Build history of the part. All positions in model axes, mm. A direction names the side the tool comes from. Coordinates: 2 decimals unless noted, no trailing zeros. Write each loop counter-clockwise with the first axis right and the second up, starting at its lowest first coordinate (ties: lowest second). Pieces come first, ordered by that corner, then holes.
```python
from build123d import *

# Parameters (mm, degrees)
F0_R     = 35.394351
F1_DEPTH = 116.078
F2_R     = 31.583321
F3_DEPTH = 108.204
F4_DEPTH = 1.016
F5_W     = 28.326623
F5_H     = 68.561267
F6_DEPTH = 66.7


with BuildPart() as f1:
    # F0 (on Front) → F1 (new body)
    with BuildSketch(Plane.XZ):
        Circle(F0_R)
    extrude(amount=F1_DEPTH)

    # F2 (on Front) → F3 (cut)
    with BuildSketch(Plane.XZ):
        Circle(F2_R)
    extrude(amount=F3_DEPTH, mode=Mode.SUBTRACT)

    # F2 (on Front) → F4 (join)
    with BuildSketch(Plane.XZ):
        Circle(F2_R)
    extrude(amount=F4_DEPTH)

    # F5 (on Top) → F6 (cut)
    with BuildSketch(Plane.XY):
        with Locations((14.163311, -59.691088)):
            Rectangle(F5_W, F5_H)
    extrude(amount=F6_DEPTH, mode=Mode.SUBTRACT)


solid = f1.part
```
1. Saw through at B-B on x = -2. List the corners of the cut face in (y, z), plus the area to 3 significant figures.
Computed values:
outline: (-116.08, -35.34) - (0, -35.34) - (0, 35.34) - (-116.08, 35.34) - close; hole (-108.2, -31.52) - (-1.02, -31.52) - (-1.02, 31.52) - (-108.2, 31.52) - close
area: 1,450 mm2
2. Saw through at A-A on z = 0. List the corners of the cut face in (x, y), plus the area to 3 significant figures.
Computed values:
outline: (-35.39, -116.08) - (35.39, -116.08) - (35.39, 0) - (-35.39, 0) - close; hole (-31.58, -108.2) - (31.58, -108.2) - (31.58, -1.02) - (-31.58, -1.02) - close
area: 1,450 mm2
3. Saw through at C-C on y = -18.5. List the corners of the cut face in (x, z), plus the area to 3 significant figures.
Computed values:
outline: circle Ø70.79 at (0, 0); hole circle Ø63.17 at (0, 0)
area: 802 mm2
4. 3-axis set-ups, long thin cutter, end or side, ignore diameter. For faces 4 (the face through (28.327, -60, 18)), 5 (the face through (0, -1.016, 0)), 6 (the face through (0, -60, 33)), 7 (the face through (0, -116.078, 0)): which of +Z, -Z, +X, -X, +Y, -Y reach the whole face in a straight line?
Computed values:
face 4: +Z
face 5: none
face 6: +Z, +X
face 7: +Z, -Z, +X, -X, -Y
5. Mould opens along Z. For faces 1 (the face through (-7.673, -57.226, -34.553)), 2 (the face through (0, 0, 0)), 3 (the face through (-6.85, -53.86, -30.83)) say: +Z half, -Z half, draft (parallel to the pull), parting line (faces both ways), or undercut.
Computed values:
face 1: parting line
face 2: draft
face 3: undercut
6. Flat gauge pins, fed straight in: pin 1 (5 mm diameter, centred on y = -13.5, z = -10.5, fed in from -X); pin 2 (1.5 mm diameter, centred on y = -64.5, z = 28, fed in from -X); pin 3 (3 mm diameter, centred on y = -26, z = -4.5, fed in from -X). Where does each tip first touch, or does it go through?
Computed values:
pin 1: stops at x = -34.48
pin 2: stops at x = -22.59
pin 3: stops at x = -35.27
7. Probe line 1 along Y through (x, z) = (15, 14); line 2 along X through (y, z) = (-61, -1); line 3 along Z through (x, y) = (-22.5, -93). List the from-to ranges inside material, lowest first.
Computed values:
line 1: y = -116.08 to -108.2, -1.02 to 0
line 2: x = -35.38 to -31.57, 31.57 to 35.38
line 3: z = -27.32 to -22.16, 22.16 to 27.32
8. Saw through at D-D on x = 13.5. List the corners of the cut face in (y, z).
Computed values:
outline: (-116.08, -32.72) - (0, -32.72) - (0, 32.72) - (-25.41, 32.72) - (-25.41, 28.55) - (-1.02, 28.55) - (-1.02, -28.55) - (-108.2, -28.55) - (-108.2, 28.55) - (-93.97, 28.55) - (-93.97, 32.72) - (-116.08, 32.72) - close
